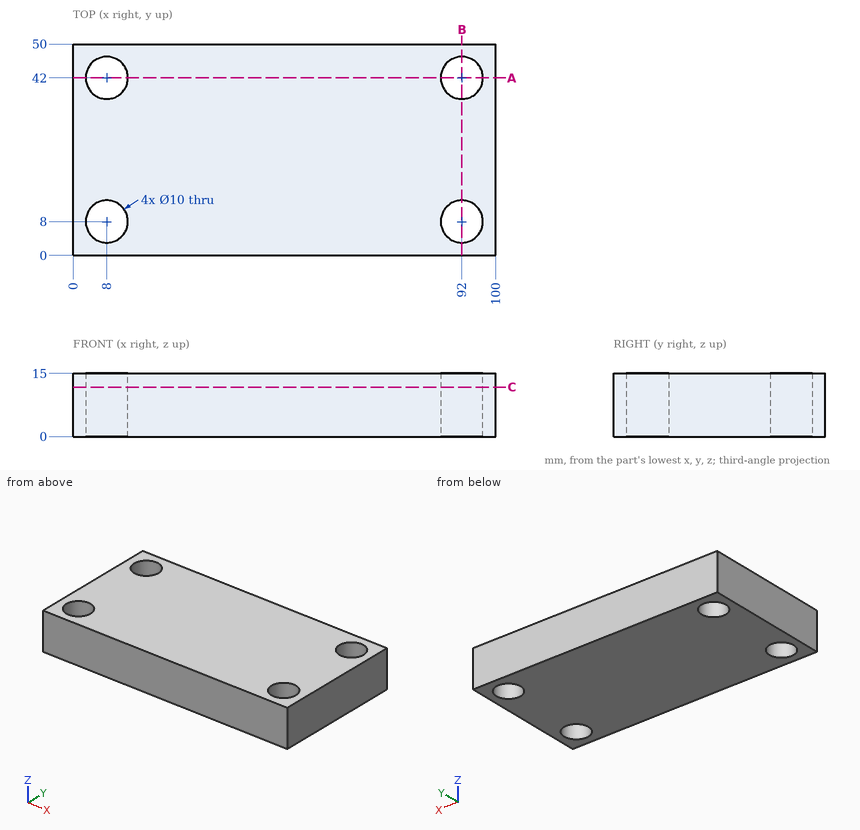
Study the drawing (mm; zero at the part's minimum x, y, z) and answer. Round coordinates to 2 decimals unless told otherwise and drop trailing zeros. Order: outer loops, then holes, each group sorted by start corner. A loop starts at its lowest first (then second) coordinate and runs counter-clockwise, first axis right, second up. Notation, with made-up numbers: (-30.5, 64) - (-20.5, 64) arc R16 cw to (-20.5, 75) - close; hole circle Ø9 at (-39.5, -17). An arc over 180 degrees is marked (long way). Use one line per item in the form item = value. Start each with the question number.
(1) The part is cut by section C-C (z = 11.75). Give the vertices of the cut face in (x, y).
(2) The part is cut by section B-B (x = 92). Give the vertices of the cut face in (y, z), then the cut area to 3 significant figures.
(3) Flat-ended cylindrical pins translate along their axes: pin 1 Ø10 at (x, y) = (51, 43.5) entering from -Z; pin 2 Ø6 at (x, y) = (92, 42) entering from -Z. Find the tip coordinate at first contact, or state that the pin passes through.
(4) Find the intervals of material crossed by line 1 along Y through (x, z) = (8, 4); line 2 along X through (y, z) = (40.5, 7.5); line 3 along X through (y, z) = (7.5, 13.25), in increasing order. Write a range as from..to.
(5) The part is cut by section A-A (y = 42). Give the vertices of the cut face in (x, z), then the cut area to 3 significant figures.
Checked values:
q1.outline = (0, 0) - (100, 0) - (100, 50) - (0, 50) - close; hole circle Ø10 at (8, 8); hole circle Ø10 at (8, 42); hole circle Ø10 at (92, 8); hole circle Ø10 at (92, 42)
q2.outline = (0, 0) - (3, 0) - (3, 15) - (0, 15) - close; (13, 0) - (37, 0) - (37, 15) - (13, 15) - close; (47, 0) - (50, 0) - (50, 15) - (47, 15) - close
q2.area = 450 mm^2
q3.pin_1 = 0
q3.pin_2 = through
q4.line_1 = 0..3, 13..37, 47..50
q4.line_2 = 0..3.23, 12.77..87.23, 96.77..100
q4.line_3 = 0..3.03, 12.97..87.03, 96.97..100
q5.outline = (0, 0) - (3, 0) - (3, 15) - (0, 15) - close; (13, 0) - (87, 0) - (87, 15) - (13, 15) - close; (97, 0) - (100, 0) - (100, 15) - (97, 15) - close
q5.area = 1,200 mm^2
